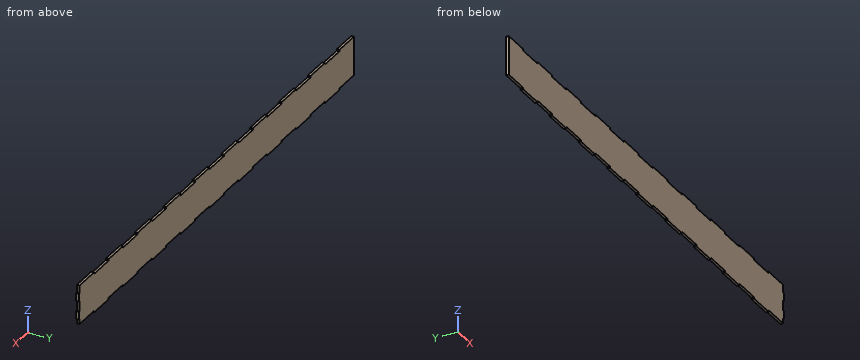
```python
from build123d import *

# Parameters (mm, degrees)
F1_DEPTH = 5


with BuildPart() as f1:
    # F0 (on Front) → F1 (new body)
    with BuildSketch(Plane.XZ):
        Polygon((-375, 35), (-425, 35), (-425, 38), (-475, 38), (-475, 35), (-475, -37), (-425, -37), (-425, -40), (-375, -40), (-375, -37), (-325, -37), (-325, -40), (-275, -40), (-275, -37), (-225, -37), (-225, -40), (-175, -40), (-175, -37), (-125, -37), (-125, -40), (-75, -40), (-75, -37), (-25, -37), (-25, -40), (25, -40), (25, -37), (75, -37), (75, -40), (125, -40), (125, -37), (175, -37), (175, -40), (225, -40), (225, -37), (275, -37), (275, -40), (325, -40), (325, -37), (375, -37), (375, -40), (425, -40), (425, -37), (475, -37), (475, -27), (478, -27), (478, -12), (475, -12), (475, 8), (478, 8), (478, 23), (475, 23), (475, 35), (475, 38), (425, 38), (425, 35), (375, 35), (375, 38), (325, 38), (325, 35), (275, 35), (275, 38), (225, 38), (225, 35), (175, 35), (175, 38), (125, 38), (125, 35), (75, 35), (75, 38), (25, 38), (25, 35), (-25, 35), (-25, 38), (-75, 38), (-75, 35), (-125, 35), (-125, 38), (-175, 38), (-175, 35), (-225, 35), (-225, 38), (-275, 38), (-275, 35), (-325, 35), (-325, 38), (-375, 38), align=None)
    extrude(amount=F1_DEPTH)


solid = f1.part
```
Work out the finished part from the listing and answer in its coordinate system (mm). Give positions to 0.01 mm unless a question says otherwise; leave off trailing zeros. Loops run counter-clockwise (first coordinate to the right, second up) from the corner with the lowest first, then second, coordinate; pieces in that order, holes last. Notation, with made-up numbers: (83.5, -14.5) -> (103.5, -14.5) arc R26 cw to (103.5, 16.5) -> close; hole circle Ø6 at (37, 85.5). An arc over 180 degrees is marked (long way). Put each result on its own line as item: value. Start each with the question number.
Item 1: Find the intervals of material crossed by L1, parallel to Z at x = 97, y = -0.55; L2, parallel to Z at x = -157.5, y = -0.4; L3, parallel to X at y = -2.8, z = 29.5, in increasing order. Write a range as [from, to].
Item 2: Each of these flat-tipped pins is pushed along its axis until it touches: P1, Ø2, axis at x = 122, z = 20, coming from the +Y side; P2, Ø3, axis at x = 334.5, y = -3, coming from the -Z side; P3, Ø2.5, axis at y = -3.5, z = -38.5, coming from the -X side; P4, Ø3, axis at x = 305, y = -0.5, coming from the +Z side. Where does it stop, or does it pass through?
Item 3: The part is cut by section A-A (x = -301). Give the vertices of the cut face in (y, z).
Answers below:
1. L1: [-40, 35]
1. L2: [-37, 38]
1. L3: [-475, 475]
2. P1: y = 0
2. P2: z = -37
2. P3: x = -425
2. P4: z = 35
3. outline: (-5, -40) -> (0, -40) -> (0, 35) -> (-5, 35) -> close
